Check sheet for the modelled part. Datum: model origin and axes. Units: mm. A direction names the side the tool comes from. Give positions to 0.01 mm unless a question says otherwise; leave off trailing zeros. Order: outer loops, then holes, each group sorted by start corner. A loop starts at its lowest first (then second) coordinate and runs counter-clockwise, first axis right, second up.
Item 1: Sectioned sample at D-D on y = 5.5. Count the separate pieces of the cut face and the enclosed holes in it, and give its area (3 significant figures).
Item 2: Sectioned sample at C-C on z = 0. Record the boundary of the cut face in (x, y), and give its area (3 significant figures).
Item 3: Sectioned sample at A-A on z = -10.25. Record the boundary of the cut face in (x, y).
Item 4: Release check for a two-part mould opening along Y. For faces 1 (the flat face through (15.5, 7, -13)), 2 (the flat face through (3.4, 11, -0.2)), 3 (the cylindrical face through (0, 4, 0)) record: released by +Y, released by -Y, zero draft, split by the parting line, or undercut.
Item 5: Access from +Z, -Z, +X, -X, +Y, -Y to the whole of each face (thin tool, end or side, straight path). Record for faces 4 (the flat face through (-3, 5, 0)), 5 (the flat face through (-18, 5, 0)), 6 (the flat face through (15.5, 7, 13)), 7 (the flat face through (4, 7, 0)).
Item 6: Gauge pin test, flat end, axial feed: P1, Ø10, axis at x = -10, z = 4.5, coming from the +Y side. Record the tip position at first contact, or that the pin passes through.
Item 7: Material ranges on line 1 along X through (y, z) = (3.5, 9.5); line 2 along X through (y, z) = (1.25, -11); line 3 along Z through (x, y) = (-4.5, 6.5), recorded low to high.
Item 8: Sectioned sample at B-B on y = 1.75. Record the boundary of the cut face in (x, z), and give its area (3 significant figures).
from build123d import *

# Parameters (mm, degrees)
BASE_REFERENCE_SKETCH_W = 15
BASE_REFERENCE_SKETCH_H = 27
BASE_EXTRUDE_DEPTH      = 3
BOSS_EXTRUDE2_START     = 3
BOSS_EXTRUDE2_DEPTH     = 8
BOSS_EXTRUDE4_START     = -3
SKETCH1_R               = 3
SKETCH1_R_2             = 1.5
BOSS_EXTRUDE4_DEPTH     = 6


with BuildPart() as part:
    # Base Reference Sketch → Base Extrude (new body)
    with BuildSketch(Plane(origin=(0, 0, 0), x_dir=(1, 0, 0), z_dir=(0, 1, 0))):
        with Locations((-10.5, 0)):
            Rectangle(BASE_REFERENCE_SKETCH_W, BASE_REFERENCE_SKETCH_H)
    extrude(amount=BASE_EXTRUDE_DEPTH)

    # Base Reference Sketch<5> → Boss-Extrude2 (add)
    with BuildSketch(Plane(origin=(0, 0, 0), x_dir=(1, 0, 0), z_dir=(0, 1, 0)).offset(BOSS_EXTRUDE2_START)):
        Polygon((-18, 13.5), (-15.5, 13.5), (-15.5, 12.5), (-17, 12.5), (-17, -12.5), (-15.5, -12.5), (-15.5, -13.5), (-18, -13.5), align=None)
        Polygon((-4, 12.5), (-4, -12.5), (-5.5, -12.5), (-5.5, -13.5), (-3, -13.5), (-3, 13.5), (-5.5, 13.5), (-5.5, 12.5), align=None)
    extrude(amount=BOSS_EXTRUDE2_DEPTH)


with BuildPart() as body_2:
    # Mirror2: mirrored copy
    add(part.part.mirror(Plane(origin=(0, 0, 0), x_dir=(0, 0, 1), z_dir=(1, 0, 0))))


with BuildPart() as part_1:
    add(part.part)

    add(body_2.part)  # Boss-Extrude4 merges body 2
    # Sketch1 → Boss-Extrude4 (add)
    with BuildSketch(Plane(origin=(0, 0, 0), x_dir=(0, 0, -1), z_dir=(1, 0, 0)).offset(BOSS_EXTRUDE4_START)):
        with Locations((0, 5.5)):
            Circle(SKETCH1_R)
        with Locations((0, 5.5)):
            Circle(SKETCH1_R_2, mode=Mode.SUBTRACT)
    extrude(amount=BOSS_EXTRUDE4_DEPTH)


solid = part_1.part
Report:
1. separate pieces: 3
1. enclosed holes: 1
1. area: 138 mm2
2. outline: (-18, 0) - (-3, 0) - (-3, 2.5) - (3, 2.5) - (3, 0) - (18, 0) - (18, 11) - (17, 11) - (17, 3) - (4, 3) - (4, 11) - (3, 11) - (3, 8.5) - (-3, 8.5) - (-3, 11) - (-4, 11) - (-4, 3) - (-17, 3) - (-17, 11) - (-18, 11) - close; hole (-3, 4) - (3, 4) - (3, 7) - (-3, 7) - close
2. area: 140 mm2
3. outline: (-18, 0) - (-3, 0) - (-3, 11) - (-4, 11) - (-4, 3) - (-17, 3) - (-17, 11) - (-18, 11) - close; (3, 0) - (18, 0) - (18, 11) - (17, 11) - (17, 3) - (4, 3) - (4, 11) - (3, 11) - close
4. face 1: zero draft
4. face 2: released by +Y
4. face 3: undercut
5. face 4: none
5. face 5: +Z, -Z, -X, +Y, -Y
5. face 6: +Z, -Z, +Y
5. face 7: +Y
6. P1: stops at y = 3
7. line 1: x = -18 to -17, -4 to -3, 3 to 4, 17 to 18
7. line 2: x = -18 to -3, 3 to 18
7. line 3: z = -13.5 to -12.5, 12.5 to 13.5
8. outline: (-18, -13.5) - (-3, -13.5) - (-3, 13.5) - (-18, 13.5) - close; (3, -13.5) - (18, -13.5) - (18, 13.5) - (3, 13.5) - close
8. area: 810 mm2
